Read the model definition and answer for the solid it produces. Units are mm, in the model's axes. A direction names the side the tool comes from. Coordinates: 2 decimals unless noted, no trailing zeros. Loops run counter-clockwise (first coordinate to the right, second up) from the corner with the lowest first, then second, coordinate; pieces in that order, holes last. Notation, with made-up numbers: (-28, 49.5) - (-16, 49.5) arc R27 ccw to (-16, 66.5) - close; hole circle Ø7 at (17, 82). An arc over 180 degrees is marked (long way). Use one line per item in the form item = value. Start each with the question number.
1) A cutting plane is placed at C-C (z = -16). Give the vertices of the cut face in (x, y), and give its area (3 significant figures).
2) Consider line 1 (X direction, y = 3, z = -10.5); line 2 (X direction, y = 4.5, z = 0); line 3 (Y direction, x = -2.3, z = -16). Determine where each line is inside the solid, lowest interval first.
3) The mould has two halves that part along Z. Classify faces 1 (the face through (1.733, 4.675, -13.856)), 2 (the face through (2, 4, -20)), 3 (the face through (-3, 4, -13)): released by +Z, released by -Z, zero draft, split by the parting line, or undercut.
4) A cutting plane is placed at D-D (x = 2.5). Give the vertices of the cut face in (y, z), and give its area (3 significant figures).
5) A cutting plane is placed at B-B (z = 0). Give the vertices of the cut face in (x, y), and give its area (3 significant figures).
6) A cutting plane is placed at A-A (y = 4). Give the vertices of the cut face in (x, z), and give its area (3 significant figures).
7) Each of these flat-tipped pins is pushed along its axis until it touches: P1, Ø2.5, axis at y = 2.5, z = -12, coming from the +X side; P2, Ø2, axis at x = -3.5, y = 2, coming from the +Z side; P3, Ø2.5, axis at y = 5.5, z = -14.5, coming from the -X side. Where does it stop, or does it pass through?
8) Which of the six approach directions +Z, -Z, +X, -X, +Y, -Y give full straight-line access (tool end or side, diameter ignored) to faces 4 (the face through (-0.5, 4, -13)), 5 (the face through (3, 4, -13)), 6 (the face through (-0.26, 3.944, 6.895))?
from build123d import *

# Parameters (mm, degrees)
BOSS_EXTRUDE1_DEPTH   = 8
F_8_CLEARANCE_HOLE1_D = 4.4958


with BuildPart() as part:
    # Sketch1 → Boss-Extrude1 (new body)
    with BuildSketch(Plane(origin=(0, 0, 0), x_dir=(1, 0, 0), z_dir=(0, 1, 0))):
        with BuildLine():
            Line((3, 6.213694553), (3, 20))
            Line((3, 20), (0.5, 20))
            Line((0.5, 20), (0.5, 5.376802024))
            ThreePointArc((0.5, 5.376802024), (0, -5.4), (-0.5, 5.376802024))
            Line((-0.5, 5.376802024), (-0.5, 20))
            Line((-0.5, 20), (-3, 20))
            Line((-3, 20), (-3, 6.213694553))
            ThreePointArc((-3, 6.213694553), (0, -6.9), (3, 6.213694553))
        make_face()
    extrude(amount=BOSS_EXTRUDE1_DEPTH)

    # #8 Clearance Hole1 (through all)
    with Locations(Plane(origin=(3, 0, 0), x_dir=(0, 0, -1), z_dir=(1, 0, 0))):
        with Locations((16, 4)):
            Hole(F_8_CLEARANCE_HOLE1_D / 2)


solid = part.part
Found:
q1.outline = (-3, 0) - (-0.5, 0) - (-0.5, 1.75) - (-3, 1.75) - close; (-3, 6.25) - (-0.5, 6.25) - (-0.5, 8) - (-3, 8) - close; (0.5, 0) - (3, 0) - (3, 1.75) - (0.5, 1.75) - close; (0.5, 6.25) - (3, 6.25) - (3, 8) - (0.5, 8) - close
q1.area = 17.5 mm^2
q2.line_1 = -3 to -0.5, 0.5 to 3
q2.line_2 = -6.9 to -5.4, 5.4 to 6.9
q2.line_3 = 0 to 1.75, 6.25 to 8
q3.face_1 = undercut
q3.face_2 = released by -Z
q3.face_3 = zero draft
q4.outline = (0, -20) - (8, -20) - (8, -4.79) - (0, -4.79) - close; (0, 4.79) - (8, 4.79) - (8, 6.43) - (0, 6.43) - close; hole circle Ø4.5 at (4, -16)
q4.area = 119 mm^2
q5.outline = (-6.9, 0) - (-5.4, 0) - (-5.4, 8) - (-6.9, 8) - close; (5.4, 0) - (6.9, 0) - (6.9, 8) - (5.4, 8) - close
q5.area = 24.0 mm^2
q6.outline = (-3, -20) - (-0.5, -20) - (-0.5, -18.25) - (-3, -18.25) - close; (-3, -13.75) - (-0.5, -13.75) - (-0.5, -5.38) arc R5.4 cw (long way) to (0.5, -5.38) - (0.5, -13.75) - (3, -13.75) - (3, -6.21) arc R6.9 ccw (long way) to (-3, -6.21) - close; (0.5, -20) - (3, -20) - (3, -18.25) - (0.5, -18.25) - close
q6.area = 101 mm^2
q7.P1 = 3
q7.P2 = 6.43
q7.P3 = -3
q8.face_4 = -Z, +Y, -Y
q8.face_5 = -Z, +X, +Y, -Y
q8.face_6 = +Y, -Y
